```python
from build123d import *

# Parameters (mm, degrees)
SKETCH1_W           = 70
SKETCH1_H           = 70
SKETCH1_R           = 2.7
BOSS_EXTRUDE1_DEPTH = 4.45
SKETCH2_R           = 22.5
CUT_EXTRUDE1_DEPTH  = 50.697107562
FILLET1_R           = 1
SKETCH4_W           = 10
SKETCH4_H           = 12
CUT_EXTRUDE3_DEPTH  = 3.5
FILLET2_R           = 1
FILLET3_R           = 1
CUT_EXTRUDE4_DEPTH  = 27.5
CUT_EXTRUDE5_DEPTH  = 14.5


with BuildPart() as part:
    # Sketch1 → Boss-Extrude1 (new body)
    with BuildSketch(Plane(origin=(0, 0, 0), x_dir=(1, 0, 0), z_dir=(0, 1, 0))):
        Rectangle(SKETCH1_W, SKETCH1_H)
        with Locations(Location((31.5, 31.5, 0), (0, 0, 270))):
            Circle(SKETCH1_R, mode=Mode.SUBTRACT)
        with Locations(Location((-31.5, 31.5, 0), (0, 0, 270))):
            Circle(SKETCH1_R, mode=Mode.SUBTRACT)
        with Locations(Location((31.5, -31.5, 0), (0, 0, 270))):
            Circle(SKETCH1_R, mode=Mode.SUBTRACT)
        with Locations(Location((-31.5, -31.5, 0), (0, 0, 270))):
            Circle(SKETCH1_R, mode=Mode.SUBTRACT)
    extrude(amount=BOSS_EXTRUDE1_DEPTH)

    # Sketch2 → Cut-Extrude1 (cut, through all)
    with BuildSketch(Plane(origin=(0, 4.45, 0), x_dir=(1, 0, 0), z_dir=(0, 1, 0))):
        with Locations(Location((0, 0, 0), (0, 0, 270))):
            Circle(SKETCH2_R)
    extrude(amount=-CUT_EXTRUDE1_DEPTH, mode=Mode.SUBTRACT)

    # Fillet1
    fillet1_edges = [part.edges().sort_by_distance(p)[0] for p in [
        (0, 4.45, -22.5),
    ]]
    fillet(fillet1_edges, radius=FILLET1_R)

    # Sketch4 → Cut-Extrude3 (cut)
    with BuildSketch(Plane(origin=(0, 4.45, 0), x_dir=(1, 0, 0), z_dir=(0, 1, 0))):
        with Locations((-30, 0)):
            Rectangle(SKETCH4_W, SKETCH4_H)
    extrude(amount=-CUT_EXTRUDE3_DEPTH, mode=Mode.SUBTRACT)

    # Fillet2
    fillet2_edges = [part.edges().sort_by_distance(p)[0] for p in [
        (0, 0, -22.5),
    ]]
    fillet(fillet2_edges, radius=FILLET2_R)

    # Fillet3
    fillet3_edges = [part.edges().sort_by_distance(p)[0] for p in [
        (-30, 4.45, -6),
        (-30, 4.45, 6),
    ]]
    fillet(fillet3_edges, radius=FILLET3_R)

    # Sketch6 → Cut-Extrude4 (cut)
    with BuildSketch(Plane.ZY.offset(35)):
        with BuildLine():
            Line((7, 4.45), (18, 4.45))
            Line((18, 4.45), (18, 0.65))
            Line((18, 0.65), (6, 0.65))
            Line((6, 0.65), (6, 3.45))
            ThreePointArc((6, 3.45), (6.292893219, 4.157106781), (7, 4.45))
        make_face()
        with BuildLine():
            Line((-7, 4.45), (-18, 4.45))
            Line((-18, 4.45), (-18, 0.65))
            Line((-18, 0.65), (-6, 0.65))
            Line((-6, 0.65), (-6, 3.45))
            ThreePointArc((-6, 3.45), (-6.292893219, 4.157106781), (-7, 4.45))
        make_face()
    extrude(amount=-CUT_EXTRUDE4_DEPTH, mode=Mode.SUBTRACT)

    # Sketch7 → Cut-Extrude5 (cut)
    with BuildSketch(Plane.ZY.offset(25)):
        with BuildLine():
            Line((7, 4.45), (-7, 4.45))
            ThreePointArc((-7, 4.45), (-6.292893219, 4.157106781), (-6, 3.45))
            Line((-6, 3.45), (-6, 0.95))
            Line((-6, 0.95), (6, 0.95))
            Line((6, 0.95), (6, 3.45))
            ThreePointArc((6, 3.45), (6.292893219, 4.157106781), (7, 4.45))
        make_face()
    extrude(amount=-CUT_EXTRUDE5_DEPTH, mode=Mode.SUBTRACT)


with BuildPart() as cut_extrude5_kept_piece:
    # of the separate pieces the step leaves, the one the design keeps (cut_extrude5_pieces_kept)
    add(part.part.solids().sort_by_distance((-35, 4.45, 18))[0])


solid = cut_extrude5_kept_piece.part
```
Can you work these out from the model? Positions are in its coordinate system, mm. A direction names the side the tool comes from. Round coordinates to 2 decimals unless told otherwise and drop trailing zeros. Loops run counter-clockwise (first coordinate to the right, second up) from the corner with the lowest first, then second, coordinate; pieces in that order, holes last. Notation, with made-up numbers: M -5.5,-30.5 L 2.5,-30.5 A19 cw 2.5,-0.5 Z; hole C 9.5,34 d8. An arc over 180 degrees is marked long. Write item = value, one per line. Start each with the question number.
(1) Suppose I cut it at B-B on z = -31.5. Write out the boundary of the cut face in (x, y), plus the area to 3 significant figures.
(2) I need wall thicknesses on line 1 along X through (y, z) = (3.2, 31.5); line 2 along Z through (x, y) = (-25, 0.8); line 3 along X through (y, z) = (0.2, 18). Which ranges of each line are inside material? Lowest first, please.
(3) Suppose I cut it at A-A on x = 0. Write out the boundary of the cut face in (y, z), plus the area to 3 significant figures.
(4) Which directions (+Z, -Z, +X, -X, +Y, -Y) give clear straight access to the entire face, cutting with the end or side of a thin tool? Please do faces 1 (the face through (22.49, 2.24, 0.7)), 2 (the face through (-28, 0.95, 0)).
(5) I'm going to push flat-ended pins straight in: P1, Ø6, axis at x = -27, z = -3, coming from the +Y side; P2, Ø6, axis at x = -27.5, z = 13.5, coming from the +Y side. Where does each tip first touch, or does it pass through?
(6) Suppose I cut it at D-D on x = 31.5. Write out the boundary of the cut face in (y, z), plus the area to 3 significant figures.
(7) Suppose I cut it at C-C on x = -31.5. Write out the boundary of the cut face in (y, z), plus the area to 3 significant figures.
Answer block:
q1.outline = M -35,0 L -34.2,0 L -34.2,4.45 L -35,4.45 Z; M -28.8,0 L 28.8,0 L 28.8,4.45 L -28.8,4.45 Z; M 34.2,0 L 35,0 L 35,4.45 L 34.2,4.45 Z
q1.area = 263 mm²
q2.line_1 = -35 to -34.2, -28.8 to 28.8, 34.2 to 35
q2.line_2 = -35 to -18, -6 to 6, 18 to 35
q2.line_3 = -35 to -14.16, 14.16 to 35
q3.outline = M 0,-35 L 4.45,-35 L 4.45,-23.5 A1 ccw 3.45,-22.5 L 1,-22.5 A1 ccw 0,-23.5 Z; M 0,23.5 A1 ccw 1,22.5 L 3.45,22.5 A1 ccw 4.45,23.5 L 4.45,35 L 0,35 Z
q3.area = 110 mm²
q4.face_1 = +Y, -Y
q4.face_2 = -X, +Y
q5.P1 = 0.95
q5.P2 = 0.65
q6.outline = M 0,-35 L 4.45,-35 L 4.45,-34.2 L 0,-34.2 Z; M 0,-28.8 L 4.45,-28.8 L 4.45,28.8 L 0,28.8 Z; M 0,34.2 L 4.45,34.2 L 4.45,35 L 0,35 Z
q6.area = 263 mm²
q7.outline = M 0,-35 L 4.45,-35 L 4.45,-34.2 L 0,-34.2 Z; M 0,-28.8 L 4.45,-28.8 L 4.45,-18 L 0.65,-18 L 0.65,-6 L 0.95,-6 L 0.95,6 L 0.65,6 L 0.65,18 L 4.45,18 L 4.45,28.8 L 0,28.8 Z; M 0,34.2 L 4.45,34.2 L 4.45,35 L 0,35 Z
q7.area = 130 mm²
